The model under review builds one solid part; all positions refer to its coordinate system, in mm. Round coordinates to 2 decimals unless told otherwise and drop trailing zeros. Answer as a JSON object with one key per item and string values. Group by question number.
1) To check wall thickness, follow probe 1 along Z at (x, y) = (-13, 2.25) (3 decimals); probe 2 along Z at (x, y) = (21.5, 1.9) (3 decimals); probe 3 along X at (y, z) = (1.7, 25). State the ranges of each line that lie inside material, in increasing order. Write a range as [from, to].
2) Insertion check: pin 1 Ø1 at (y, z) = (2.5, 21) entering from +X; pin 2 Ø1.9 at (y, z) = (2, 59) entering from +X; pin 3 Ø1 at (y, z) = (1.5, 17) entering from -X. Each pin has a flat end and moves straight along its axis. Give the tip position at first contact, or say it passes through.
3) We need section A-A, the plane x = 18.5. Count the separate pieces of the cut face and the enclosed holes in it, then the cut area to 3 significant figures.
from build123d import *

# Parameters (mm, degrees)
SKETCH1_R                   = 76.1
BOSS_EXTRUDE1_DEPTH         = 3.175
SKETCH3_W                   = 15.4
SKETCH3_H                   = 3.175
CUT_EXTRUDE1_DEPTH          = 108.66847554
SKETCH4_R                   = 0.5
CUT_EXTRUDE2_DEPTH          = 108.66847554
SKETCH_PATTERN1_DEPTH       = 3.175
CIRPATTERN1_COUNT           = 4
CIRPATTERN1_COPY_1_SKETCH_R = 0.5
CIRPATTERN1_COPY_1_DEPTH    = 108.66847554
CIRPATTERN1_COPY_2_SKETCH_R = 0.5
CIRPATTERN1_COPY_2_DEPTH    = 108.66847554
CIRPATTERN1_COPY_3_SKETCH_R = 0.5
CIRPATTERN1_COPY_3_DEPTH    = 108.66847554
CIRPATTERN1_COPY_4_DEPTH    = 3.175
CIRPATTERN1_COPY_5_DEPTH    = 3.175
CIRPATTERN1_COPY_6_DEPTH    = 3.175
SKETCH2_W                   = 100
SKETCH2_H                   = 100
CUT_EXTRUDE3_DEPTH          = 0.0001
SKETCH7_W                   = 8.5
SKETCH7_H                   = 8.5
CUT_EXTRUDE4_DEPTH          = 0.0001


# Read off the part's stored shape, not the designer's step: Sketch-Pattern1
with BuildPart() as part:
    # Sketch1 → Boss-Extrude1 (new body)
    with BuildSketch(Plane(origin=(0, 0, 0), x_dir=(1, 0, 0), z_dir=(0, 1, 0))):
        with Locations(Location((0, 0, 0), (0, 0, 270))):
            Circle(SKETCH1_R)
    extrude(amount=BOSS_EXTRUDE1_DEPTH)

    # Sketch3 → Cut-Extrude1 (cut, symmetric)
    with BuildSketch(Plane(origin=(0, 3.175, 0), x_dir=(1, 0, 0), z_dir=(0, 1, 0))):
        with Locations((-17.7, 58.6875)):
            Rectangle(SKETCH3_W, SKETCH3_H)
        with Locations((17.7, 58.6875)):
            Rectangle(SKETCH3_W, SKETCH3_H)
    cut_extrude1 = extrude(amount=CUT_EXTRUDE1_DEPTH, both=True, mode=Mode.SUBTRACT)

    # Sketch4 → Cut-Extrude2 (cut, symmetric)
    with BuildSketch(Plane(origin=(0, 3.175, 0), x_dir=(1, 0, 0), z_dir=(0, 1, 0))):
        with Locations((-25.046446609, 59.921446609)):
            Circle(SKETCH4_R)
        with Locations((-25.046446609, 57.453553391)):
            Circle(SKETCH4_R)
    cut_extrude2 = extrude(amount=CUT_EXTRUDE2_DEPTH, both=True, mode=Mode.SUBTRACT)

    # Sketch-Pattern1 outline → Sketch-Pattern1 (cut)
    with BuildSketch(Plane(origin=(0, 0, 0), x_dir=(1, 0, 0), z_dir=(0, 1, 0))):
        with BuildLine():
            Line((10, 60.275), (10.707106781, 60.275))
            ThreePointArc((10.707106781, 60.275), (10.353553391, 60.421446609), (10, 60.275))
        make_face()
        with BuildLine():
            Line((10.707106781, 57.1), (10, 57.1))
            ThreePointArc((10, 57.1), (10.353553391, 56.953553391), (10.707106781, 57.1))
        make_face()
        with BuildLine():
            Line((10, 57.1), (10, 57.807106781))
            ThreePointArc((10, 57.807106781), (9.853553391, 57.453553391), (10, 57.1))
        make_face()
        with BuildLine():
            Line((10, 59.567893219), (10, 60.275))
            ThreePointArc((10, 60.275), (9.853553391, 59.921446609), (10, 59.567893219))
        make_face()
    sketch_pattern1 = extrude(amount=SKETCH_PATTERN1_DEPTH, mode=Mode.SUBTRACT)

    # Mirror1: Cut-Extrude2, Sketch-Pattern1 across plane
    add(cut_extrude2.mirror(Plane(origin=(0, 0, 0), x_dir=(0, 0, 1), z_dir=(1, 0, 0))), mode=Mode.SUBTRACT)
    add(sketch_pattern1.mirror(Plane(origin=(0, 0, 0), x_dir=(0, 0, 1), z_dir=(1, 0, 0))), mode=Mode.SUBTRACT)

    # CirPattern1: Cut-Extrude1, Cut-Extrude2, Sketch-Pattern1 ×4 about axis
    cirpattern1_axis = Axis((0, 0, 0), (0, 1, 0))
    add([cut_extrude1.rotate(cirpattern1_axis, i * 360 / CIRPATTERN1_COUNT) for i in range(1, CIRPATTERN1_COUNT)], mode=Mode.SUBTRACT)
    add([cut_extrude2.rotate(cirpattern1_axis, i * 360 / CIRPATTERN1_COUNT) for i in range(1, CIRPATTERN1_COUNT)], mode=Mode.SUBTRACT)
    add([sketch_pattern1.rotate(cirpattern1_axis, i * 360 / CIRPATTERN1_COUNT) for i in range(1, CIRPATTERN1_COUNT)], mode=Mode.SUBTRACT)

    # CirPattern1 copy 1 sketch → CirPattern1 copy 1 (cut, symmetric)
    with BuildSketch(Plane.ZX.offset(3.175)):
        with Locations((-25.046446609, -59.921446609)):
            Circle(CIRPATTERN1_COPY_1_SKETCH_R)
        with Locations((-25.046446609, -57.453553391)):
            Circle(CIRPATTERN1_COPY_1_SKETCH_R)
    extrude(amount=CIRPATTERN1_COPY_1_DEPTH, both=True, mode=Mode.SUBTRACT)

    # CirPattern1 copy 2 sketch → CirPattern1 copy 2 (cut, symmetric)
    with BuildSketch(Plane(origin=(0, 3.175, 0), x_dir=(1, 0, 0), z_dir=(0, 1, 0))):
        with Locations((-25.046446609, -59.921446609)):
            Circle(CIRPATTERN1_COPY_2_SKETCH_R)
        with Locations((-25.046446609, -57.453553391)):
            Circle(CIRPATTERN1_COPY_2_SKETCH_R)
    extrude(amount=CIRPATTERN1_COPY_2_DEPTH, both=True, mode=Mode.SUBTRACT)

    # CirPattern1 copy 3 sketch → CirPattern1 copy 3 (cut, symmetric)
    with BuildSketch(Plane(origin=(0, 3.175, 0), x_dir=(0, 0, -1), z_dir=(0, 1, 0))):
        with Locations((-25.046446609, -59.921446609)):
            Circle(CIRPATTERN1_COPY_3_SKETCH_R)
        with Locations((-25.046446609, -57.453553391)):
            Circle(CIRPATTERN1_COPY_3_SKETCH_R)
    extrude(amount=CIRPATTERN1_COPY_3_DEPTH, both=True, mode=Mode.SUBTRACT)

    # CirPattern1 copy 4 sketch → CirPattern1 copy 4 (cut)
    with BuildSketch(Plane.ZX):
        with BuildLine():
            Line((10, -60.275), (10.707106781, -60.275))
            ThreePointArc((10.707106781, -60.275), (10.353553391, -60.421446609), (10, -60.275))
        make_face()
        with BuildLine():
            Line((10.707106781, -57.1), (10, -57.1))
            ThreePointArc((10, -57.1), (10.353553391, -56.953553391), (10.707106781, -57.1))
        make_face()
        with BuildLine():
            Line((10, -57.1), (10, -57.807106781))
            ThreePointArc((10, -57.807106781), (9.853553391, -57.453553391), (10, -57.1))
        make_face()
        with BuildLine():
            Line((10, -59.567893219), (10, -60.275))
            ThreePointArc((10, -60.275), (9.853553391, -59.921446609), (10, -59.567893219))
        make_face()
    extrude(amount=CIRPATTERN1_COPY_4_DEPTH, mode=Mode.SUBTRACT)

    # CirPattern1 copy 5 sketch → CirPattern1 copy 5 (cut)
    with BuildSketch(Plane(origin=(0, 0, 0), x_dir=(1, 0, 0), z_dir=(0, 1, 0))):
        with BuildLine():
            Line((10, -60.275), (10.707106781, -60.275))
            ThreePointArc((10.707106781, -60.275), (10.353553391, -60.421446609), (10, -60.275))
        make_face()
        with BuildLine():
            Line((10.707106781, -57.1), (10, -57.1))
            ThreePointArc((10, -57.1), (10.353553391, -56.953553391), (10.707106781, -57.1))
        make_face()
        with BuildLine():
            Line((10, -57.1), (10, -57.807106781))
            ThreePointArc((10, -57.807106781), (9.853553391, -57.453553391), (10, -57.1))
        make_face()
        with BuildLine():
            Line((10, -59.567893219), (10, -60.275))
            ThreePointArc((10, -60.275), (9.853553391, -59.921446609), (10, -59.567893219))
        make_face()
    extrude(amount=CIRPATTERN1_COPY_5_DEPTH, mode=Mode.SUBTRACT)

    # CirPattern1 copy 6 sketch → CirPattern1 copy 6 (cut)
    with BuildSketch(Plane(origin=(0, 0, 0), x_dir=(0, 0, -1), z_dir=(0, 1, 0))):
        with BuildLine():
            Line((10, -60.275), (10.707106781, -60.275))
            ThreePointArc((10.707106781, -60.275), (10.353553391, -60.421446609), (10, -60.275))
        make_face()
        with BuildLine():
            Line((10.707106781, -57.1), (10, -57.1))
            ThreePointArc((10, -57.1), (10.353553391, -56.953553391), (10.707106781, -57.1))
        make_face()
        with BuildLine():
            Line((10, -57.1), (10, -57.807106781))
            ThreePointArc((10, -57.807106781), (9.853553391, -57.453553391), (10, -57.1))
        make_face()
        with BuildLine():
            Line((10, -59.567893219), (10, -60.275))
            ThreePointArc((10, -60.275), (9.853553391, -59.921446609), (10, -59.567893219))
        make_face()
    extrude(amount=CIRPATTERN1_COPY_6_DEPTH, mode=Mode.SUBTRACT)

    # Sketch2 → Cut-Extrude3 (cut)
    with BuildSketch(Plane(origin=(0, 3.175, 0), x_dir=(1, 0, 0), z_dir=(0, 1, 0))):
        Rectangle(SKETCH2_W, SKETCH2_H)
    extrude(amount=-CUT_EXTRUDE3_DEPTH, mode=Mode.SUBTRACT)

    # Sketch7 → Cut-Extrude4 (cut)
    with BuildSketch(Plane(origin=(0, 3.1749, 0), x_dir=(1, 0, 0), z_dir=(0, 1, 0))):
        with Locations((-45.75, 45.75)):
            Rectangle(SKETCH7_W, SKETCH7_H)
        with Locations((45.75, 45.75)):
            Rectangle(SKETCH7_W, SKETCH7_H)
        with Locations((45.75, -45.75)):
            Rectangle(SKETCH7_W, SKETCH7_H)
        with Locations((-45.75, -45.75)):
            Rectangle(SKETCH7_W, SKETCH7_H)
    extrude(amount=-CUT_EXTRUDE4_DEPTH, mode=Mode.SUBTRACT)


solid = part.part
Here are the results:
{
 "1": {"probe 1": "z = [-74.981, -60.275], [-57.1, 57.1], [60.275, 74.981]", "probe 2": "z = [-73, -60.275], [-57.1, 57.1], [60.275, 73]", "probe 3": "x = [-71.88, -60.42], [-56.96, 56.96], [60.42, 71.88]"},
 "2": {"pin 1": "stops at x = 73.29", "pin 2": "stops at x = 49.21", "pin 3": "stops at x = -74.29"},
 "3": {"separate pieces": "3", "enclosed holes": "0", "area": "449 mm^2"}
}
